```python
from build123d import *

# Parameters (mm, degrees)
F1_DEPTH = 20
F2_START = 15
F2_DEPTH = 10
F4_DEPTH = 2.000000095


with BuildPart() as f1:
    # F0 (on Top) → F1 (new body)
    with BuildSketch(Plane.XY):
        with BuildLine():
            Line((9, 0), (-11, 0))
            ThreePointArc((-11, 0), (0, -11), (11, 0))
            ThreePointArc((11, 0), (10.4880884817, 3.3166247904), (9, 6.3245553203))
            Line((9, 6.3245553203), (9, 0))
        make_face()
        with BuildLine():
            ThreePointArc((9, 6.3245553203), (-3.3166247904, 10.4880884817), (-11, 0))
            Line((-11, 0), (9, 0))
            Line((9, 0), (9, 6.3245553203))
        make_face()
    extrude(amount=F1_DEPTH)

    # F0 (on Top) → F2 (join)
    with BuildSketch(Plane.XY.offset(F2_START)):
        with BuildLine():
            Line((9, 0), (-11, 0))
            ThreePointArc((-11, 0), (0, -11), (11, 0))
            ThreePointArc((11, 0), (10.4880884817, 3.3166247904), (9, 6.3245553203))
            Line((9, 6.3245553203), (9, 0))
        make_face()
        with BuildLine():
            Line((-11, 100), (-11, 0))
            ThreePointArc((-11, 0), (-3.3166247904, 10.4880884817), (9, 6.3245553203))
            Line((9, 6.3245553203), (9, 100))
            Line((9, 100), (-11, 100))
        make_face()
        with BuildLine():
            ThreePointArc((9, 6.3245553203), (-3.3166247904, 10.4880884817), (-11, 0))
            Line((-11, 0), (9, 0))
            Line((9, 0), (9, 6.3245553203))
        make_face()
    extrude(amount=F2_DEPTH)

    # F3 (on Top) → F4 (cut)
    with BuildSketch(Plane.XY):
        with BuildLine():
            Line((9.0059984515, -8.6684480671), (7.3840666789, -4.2631928848))
            Line((7.3840666789, -4.2631928848), (12.0100954632, -3.4651994118))
            ThreePointArc((12.0100954632, -3.4651994118), (12.3769178977, -1.7498295216), (12.5, 0))
            ThreePointArc((12.5, 0), (12.3769178977, 1.7498295216), (12.0100954632, 3.4651994118))
            Line((12.0100954632, 3.4651994118), (7.3840666789, 4.2631928848))
            Line((7.3840666789, 4.2631928848), (9.0059984515, 8.6684480671))
            ThreePointArc((9.0059984515, 8.6684480671), (6.25, 10.8253175473), (3.0040970118, 12.133647479))
            Line((3.0040970118, 12.133647479), (0, 8.5263857696))
            Line((0, 8.5263857696), (-3.0040970118, 12.133647479))
            ThreePointArc((-3.0040970118, 12.133647479), (-6.25, 10.8253175473), (-9.0059984515, 8.6684480671))
            Line((-9.0059984515, 8.6684480671), (-7.3840666789, 4.2631928848))
            Line((-7.3840666789, 4.2631928848), (-12.0100954632, 3.4651994118))
            ThreePointArc((-12.0100954632, 3.4651994118), (-12.5, 0), (-12.0100954632, -3.4651994118))
            Line((-12.0100954632, -3.4651994118), (-7.3840666789, -4.2631928848))
            Line((-7.3840666789, -4.2631928848), (-9.0059984515, -8.6684480671))
            ThreePointArc((-9.0059984515, -8.6684480671), (-6.25, -10.8253175473), (-3.0040970118, -12.133647479))
            Line((-3.0040970118, -12.133647479), (0, -8.5263857696))
            Line((0, -8.5263857696), (3.0040970118, -12.133647479))
            ThreePointArc((3.0040970118, -12.133647479), (6.25, -10.8253175473), (9.0059984515, -8.6684480671))
        make_face()
    extrude(amount=F4_DEPTH, mode=Mode.SUBTRACT)


solid = f1.part
```
Geometry: final body of the model. Coordinates: model frame, mm. A direction names the side the tool comes from. Give positions to 0.01 mm unless a question says otherwise; leave off trailing zeros. Loops run counter-clockwise (first coordinate to the right, second up) from the corner with the lowest first, then second, coordinate; pieces in that order, holes last. Notation, with made-up numbers: (14, -14) -> (55, -14) arc R12 cw to (55, -4) -> close; hole circle Ø1 at (11.25, -29). An arc over 180 degrees is marked (long way). Return JSON: item names as keys, results as strings.
Item 1: Section B-B, the plane z = 7.75. Output: boundary loops of the cut face in (x, y).
Filled in:
{"outline": "circle Ø22 at (0, 0)"}
Item 2: Pin query (flat end, axial travel): P1, Ø11, axis at x = 1.5, y = 3, coming from the -Z side; P2, Ø5, axis at y = 52, z = 20.5, coming from the +X side; P3, Ø3, axis at x = -3, z = 21.5, coming from the -Y side. Return the tip coordinate at first contact, or that it passes through.
Filled in:
{"P1": "z = 2", "P2": "x = 9", "P3": "y = -10.9"}
Item 3: Access query for faces 1 (the flat face through (9, 53, 20)), 2 (the flat face through (0.97, 9.69, 0.99)), 3 (the flat face through (7.895, 5.651, 0.986)), 4 (the cylindrical face through (4.22, -10.16, 12.32)). Directions: +Z, -Z, +X, -X, +Y, -Y. A direction counts if a zero-diameter tool reaches every point of the face in a straight line with its end or side. Return the directions, or none.
Filled in:
{"face 1": "+Z, -Z, +X, +Y", "face 2": "-Z, +X", "face 3": "-Z, +Y", "face 4": "-Z"}
Item 4: Mould query, pull axis X, two halves, no side actions, for faces 5 (the flat face through (-0.97, -9.69, 0.99)), 6 (the flat face through (-9, -5, 0)), 7 (the flat face through (-7.91, 5.69, 0.99)). Classes: released by +X, released by -X, zero draft, split by the parting line, or undercut.
Filled in:
{"face 5": "released by -X", "face 6": "zero draft", "face 7": "undercut"}
Item 5: Section A-A, the plane y = 89.5. Output: boundary loops of the cut face in (x, z).
Filled in:
{"outline": "(-11, 15) -> (9, 15) -> (9, 25) -> (-11, 25) -> close"}
Item 6: Line query: line 1 (Z direction, x = 6.5, y = -2.5); line 2 (Z direction, x = -1.25, y = 50); line 3 (X direction, y = 73.5, z = 22.5). Output: solid intervals per line, ascending.
Filled in:
{"line 1": "2 to 25", "line 2": "15 to 25", "line 3": "-11 to 9"}
